For this review, take the finished solid that the model builds, in its own axes (mm). A direction names the side the tool comes from. Give positions to 0.01 mm unless a question says otherwise; leave off trailing zeros. Order: outer loops, then holes, each group sorted by start corner. A loop starts at its lowest first (then second) coordinate and runs counter-clockwise, first axis right, second up. Notation, with made-up numbers: M 63,-23 L 81,-23 A29 ccw 81,-3 Z; hole C 6.5,-8 d1. An arc over 180 degrees is marked long. Use CSV: the item, a comma, the result in double quotes. Start each with the question number.
(1) Wall thickness on L1, parallel to X at y = -6.4, z = 8; L2, parallel to X at y = 14.6, z = 88; L3, parallel to Z at x = -3.25, y = 1.5: over which ranges is each line inside the solid? List them lowest first. Write a range as from..to.
(2) Draft analysis for pull direction X (two halves, no side actions). For faces 6 (the face through (8.936, 12.535, 96.741)), 7 (the face through (-5.582, 11.521, 94.474)), 8 (the face through (-2, -7.5, 10)), state which applies: pulls with the +X half, pulls with the -X half, needs draft (parallel to the pull), parting line crosses it, or undercut.
(3) Tool access review of faces 1 (the face through (3, -2, 75.5)), 2 (the face through (0.1, 12, 85.5)), 3 (the face through (4.61, -5.34, 7.39)), 4 (the face through (1.5, 5, 81)), 5 (the face through (-0.2, 10.2, 70.5)): name each direction out of +Z, -Z, +X, -X, +Y, -Y from which nothing blocks a thin tool from reaching the whole face with its end or side.
(4) Clearance check with flat-ended pins moving along their axes: P1, Ø5, axis at y = 3.5, z = 13, coming from the +X side; P2, Ø1, axis at x = -9.5, z = 70.5, coming from the -Y side; P3, Ø1, axis at y = -6.5, z = 77, coming from the +X side; P4, Ø12.5, axis at x = -3.5, y = 7, coming from the -Z side. State where each tip first meets the part, or that it passes through.
(5) Consider section A-A (z = 8). Write out the cut boundary in (x, y).
(6) Consider section B-B (y = 0). Write out the cut boundary in (x, z).
```python
from build123d import *

# Parameters (mm, degrees)
SKETCH1_R                           = 5
BOSS_EXTRUDE1_DEPTH                 = 70.5
SKETCH3_W                           = 25
SKETCH3_H                           = 30
BOSS_EXTRUDE3_DEPTH                 = 5
SKETCH4_W                           = 25
SKETCH4_H                           = 5
BOSS_EXTRUDE4_DEPTH                 = 25
FILLET3_R                           = 12.5
CUT_EXTRUDE1_REACH                  = 107.624
SKETCH6_R                           = 1.65
SKETCH6_3_R                         = 10
SKETCH6_3_R_2                       = 1.65
SKETCH6_3_R_3                       = 2.5
CUT_EXTRUDE2_DEPTH                  = 2
SKETCH6_4_R                         = 2.5
CUT_EXTRUDE3_DEPTH                  = 4
FILLET4_R                           = 5
CUT_EXTRUDE4_REACH                  = 104.379
CUT_EXTRUDE4_END_RADIUS             = 5
SKETCH7_R                           = 2.65
CUT_EXTRUDE4_DIRECTION_2_REACH      = 104.379
CUT_EXTRUDE4_DIRECTION_2_END_RADIUS = 5
BOSS_EXTRUDE6_DEPTH                 = 7.5
BOSS_EXTRUDE6_DEPTH_BACK            = 7.5
SKETCH7_3_R                         = 4.65
SKETCH7_3_R_2                       = 2.65
BOSS_EXTRUDE7_DEPTH                 = 1.5
BOSS_EXTRUDE7_DEPTH_BACK            = 1.5


with BuildPart() as part:
    # Sketch1 → Boss-Extrude1 (new body)
    with BuildSketch(Plane(origin=(0, 0, 0), x_dir=(0, 1, 0), z_dir=(0, 0, 1))):
        with Locations(Location((0, 0, 0), (0, 0, 270))):
            Circle(SKETCH1_R)
    extrude(amount=BOSS_EXTRUDE1_DEPTH)

    # Sketch3 → Boss-Extrude3 (add)
    with BuildSketch(Plane.XY.offset(70.5)):
        Rectangle(SKETCH3_W, SKETCH3_H)
    extrude(amount=BOSS_EXTRUDE3_DEPTH)

    # Sketch4 → Boss-Extrude4 (add)
    with BuildSketch(Plane.XY.offset(75.5)):
        with Locations((0, 12.5)):
            Rectangle(SKETCH4_W, SKETCH4_H)
    extrude(amount=BOSS_EXTRUDE4_DEPTH)

    # Fillet3
    fillet3_edges = [part.edges().sort_by_distance(p)[0] for p in [
        (12.5, 12.5, 100.5),
        (-12.5, 12.5, 100.5),
        (-12.5, -15, 73),
        (12.5, -15, 73),
    ]]
    fillet(fillet3_edges, radius=FILLET3_R - 0.0001)  # a hair under: the kernel refuses the full size

    # Sketch6 → Cut-Extrude1 (cut, up to next)
    with BuildSketch(Plane(origin=(0, 15, 0), x_dir=(-1, 0, 0), z_dir=(0, 1, 0)), mode=Mode.PRIVATE) as cut_extrude1_sk1:
        with Locations(Location((-4.949747468, 92.949747468, 0), (0, 0, 90))):
            Circle(SKETCH6_R)
    cut_extrude1_tool1 = extrude(cut_extrude1_sk1.sketch, amount=-CUT_EXTRUDE1_REACH, mode=Mode.PRIVATE) & part.part
    # Sketch6 → Cut-Extrude1 (cut, up to next)
    with BuildSketch(Plane(origin=(0, 15, 0), x_dir=(-1, 0, 0), z_dir=(0, 1, 0)), mode=Mode.PRIVATE) as cut_extrude1_sk2:
        with Locations(Location((4.949747468, 92.949747468, 0), (0, 0, 90))):
            Circle(SKETCH6_R)
    cut_extrude1_tool2 = extrude(cut_extrude1_sk2.sketch, amount=-CUT_EXTRUDE1_REACH, mode=Mode.PRIVATE) & part.part
    # Sketch6 → Cut-Extrude1 (cut, up to next)
    with BuildSketch(Plane(origin=(0, 15, 0), x_dir=(-1, 0, 0), z_dir=(0, 1, 0)), mode=Mode.PRIVATE) as cut_extrude1_sk3:
        with Locations(Location((-4.949747468, 83.050252532, 0), (0, 0, 90))):
            Circle(SKETCH6_R)
    cut_extrude1_tool3 = extrude(cut_extrude1_sk3.sketch, amount=-CUT_EXTRUDE1_REACH, mode=Mode.PRIVATE) & part.part
    # Sketch6 → Cut-Extrude1 (cut, up to next)
    with BuildSketch(Plane(origin=(0, 15, 0), x_dir=(-1, 0, 0), z_dir=(0, 1, 0)), mode=Mode.PRIVATE) as cut_extrude1_sk4:
        with Locations(Location((4.949747468, 83.050252532, 0), (0, 0, 90))):
            Circle(SKETCH6_R)
    cut_extrude1_tool4 = extrude(cut_extrude1_sk4.sketch, amount=-CUT_EXTRUDE1_REACH, mode=Mode.PRIVATE) & part.part
    add(cut_extrude1_tool1.solids().sort_by_distance((4.949747, 15, 92.949747))[0], mode=Mode.SUBTRACT)
    add(cut_extrude1_tool2.solids().sort_by_distance((-4.949747, 15, 92.949747))[0], mode=Mode.SUBTRACT)
    add(cut_extrude1_tool3.solids().sort_by_distance((4.949747, 15, 83.050253))[0], mode=Mode.SUBTRACT)
    add(cut_extrude1_tool4.solids().sort_by_distance((-4.949747, 15, 83.050253))[0], mode=Mode.SUBTRACT)

    # Sketch6<3> → Cut-Extrude2 (cut)
    # profile 1 of 6: a face of its own
    with BuildSketch(Plane(origin=(0, 15, 0), x_dir=(-1, 0, 0), z_dir=(0, 1, 0))):
        with Locations(Location((0, 88, 0), (0, 0, 90))):
            Circle(SKETCH6_3_R)
        with Locations(Location((4.949747468, 83.050252532, 0), (0, 0, 90))):
            Circle(SKETCH6_3_R_2, mode=Mode.SUBTRACT)
        with Locations(Location((-4.949747468, 83.050252532, 0), (0, 0, 90))):
            Circle(SKETCH6_3_R_2, mode=Mode.SUBTRACT)
        with Locations(Location((4.949747468, 92.949747468, 0), (0, 0, 90))):
            Circle(SKETCH6_3_R_2, mode=Mode.SUBTRACT)
        with Locations(Location((-4.949747468, 92.949747468, 0), (0, 0, 90))):
            Circle(SKETCH6_3_R_2, mode=Mode.SUBTRACT)
        with Locations((0, 88)):
            Circle(SKETCH6_3_R_3, mode=Mode.SUBTRACT)
    # profile 2 of 6: a face of its own
    with BuildSketch(Plane(origin=(0, 15, 0), x_dir=(-1, 0, 0), z_dir=(0, 1, 0))):
        with Locations(Location((4.949747468, 92.949747468, 0), (0, 0, 90))):
            Circle(SKETCH6_3_R_2)
    # profile 3 of 6: a face of its own
    with BuildSketch(Plane(origin=(0, 15, 0), x_dir=(-1, 0, 0), z_dir=(0, 1, 0))):
        with Locations(Location((-4.949747468, 92.949747468, 0), (0, 0, 90))):
            Circle(SKETCH6_3_R_2)
    # profile 4 of 6: a face of its own
    with BuildSketch(Plane(origin=(0, 15, 0), x_dir=(-1, 0, 0), z_dir=(0, 1, 0))):
        with Locations(Location((-4.949747468, 83.050252532, 0), (0, 0, 90))):
            Circle(SKETCH6_3_R_2)
    # profile 5 of 6: a face of its own
    with BuildSketch(Plane(origin=(0, 15, 0), x_dir=(-1, 0, 0), z_dir=(0, 1, 0))):
        with Locations(Location((4.949747468, 83.050252532, 0), (0, 0, 90))):
            Circle(SKETCH6_3_R_2)
    # profile 6 of 6: a face of its own
    with BuildSketch(Plane(origin=(0, 15, 0), x_dir=(-1, 0, 0), z_dir=(0, 1, 0))):
        with Locations((0, 88)):
            Circle(SKETCH6_3_R_3)
    extrude(amount=-CUT_EXTRUDE2_DEPTH, mode=Mode.SUBTRACT)

    # Sketch6<4> → Cut-Extrude3 (cut)
    with BuildSketch(Plane(origin=(0, 15, 0), x_dir=(-1, 0, 0), z_dir=(0, 1, 0))):
        with Locations(Location((0, 88, 0), (0, 0, 90))):
            Circle(SKETCH6_4_R)
    extrude(amount=-CUT_EXTRUDE3_DEPTH, mode=Mode.SUBTRACT)

    # Fillet4
    fillet4_edges = [part.edges().sort_by_distance(p)[0] for p in [
        (-5, 0, 70.5),
    ]]
    fillet(fillet4_edges, radius=FILLET4_R)

    # Cut-Extrude4: up to this cylinder (the profile starts inside it)
    cut_extrude4_end = Plane(origin=(0, 0, 8), z_dir=(0, 0, -1)) * Cylinder(CUT_EXTRUDE4_END_RADIUS, 219.758, mode=Mode.PRIVATE)
    # Sketch7 → Cut-Extrude4 (cut, up to the surface)
    with BuildSketch(Plane(origin=(0, 0, 0), x_dir=(-1, 0, 0), z_dir=(0, 1, 0)), mode=Mode.PRIVATE) as cut_extrude4_sk1:
        with Locations(Location((0, 8, 0), (0, 0, 270))):
            Circle(SKETCH7_R)
    cut_extrude4_tool1 = extrude(cut_extrude4_sk1.sketch, amount=-CUT_EXTRUDE4_REACH, mode=Mode.PRIVATE) & cut_extrude4_end
    add(cut_extrude4_tool1.solids().sort_by_distance((0, 0, 8))[0], mode=Mode.SUBTRACT)

    # Cut-Extrude4 direction 2: up to this cylinder (the profile starts inside it)
    cut_extrude4_direction_2_end = Plane(origin=(0, 0, 8), z_dir=(0, 0, -1)) * Cylinder(CUT_EXTRUDE4_DIRECTION_2_END_RADIUS, 219.758, mode=Mode.PRIVATE)
    # Sketch7 → Cut-Extrude4 direction 2 (cut, up to the surface)
    with BuildSketch(Plane(origin=(0, 0, 0), x_dir=(-1, 0, 0), z_dir=(0, 1, 0)), mode=Mode.PRIVATE) as cut_extrude4_direction_2_sk1:
        with Locations(Location((0, 8, 0), (0, 0, 270))):
            Circle(SKETCH7_R)
    cut_extrude4_direction_2_tool1 = extrude(cut_extrude4_direction_2_sk1.sketch, amount=CUT_EXTRUDE4_DIRECTION_2_REACH, mode=Mode.PRIVATE) & cut_extrude4_direction_2_end
    add(cut_extrude4_direction_2_tool1.solids().sort_by_distance((0, 0, 8))[0], mode=Mode.SUBTRACT)

    # Sketch7<3> → Boss-Extrude6 (add, two sides: drawn at the far end of the back side and taken through both)
    with BuildSketch(Plane(origin=(0, 0, 0), x_dir=(-1, 0, 0), z_dir=(0, 1, 0)).offset(-BOSS_EXTRUDE6_DEPTH_BACK)):
        with Locations(Location((0, 8, 0), (0, 0, 90))):
            Circle(SKETCH7_3_R)
        with Locations(Location((0, 8, 0), (0, 0, 270))):
            Circle(SKETCH7_3_R_2, mode=Mode.SUBTRACT)
    extrude(amount=BOSS_EXTRUDE6_DEPTH + BOSS_EXTRUDE6_DEPTH_BACK)

    # Sketch9 → Boss-Extrude7 (add, two sides: drawn at the far end of the back side and taken through both)
    with BuildSketch(Plane(origin=(0, 0, 0), x_dir=(0, -1, 0), z_dir=(-1, 0, 0)).offset(-BOSS_EXTRUDE7_DEPTH_BACK)):
        Polygon((-10, 94.25), (8.75, 75.5), (-10, 75.5), align=None)
    extrude(amount=BOSS_EXTRUDE7_DEPTH + BOSS_EXTRUDE7_DEPTH_BACK)


solid = part.part
```
Check result:
1,L1,"x = -4.65..-2.65, 2.65..4.65"
1,L2,"x = -12.5..-10, 10..12.5"
1,L3,"z = 0..75.5"
2,face 6,"pulls with the +X half"
2,face 7,"undercut"
2,face 8,"needs draft"
3,face 1,"+Z, -Y"
3,face 2,"+Y"
3,face 3,"-Y"
3,face 4,"+Z, +X, -Y"
3,face 5,"-Z"
4,P1,"stops at x = 4.9"
4,P2,"stops at y = -11.17"
4,P3,"stops at x = 1.5"
4,P4,"stops at z = 0"
5,outline,"M -4.65,-7.5 L -2.65,-7.5 L -2.65,7.5 L -4.65,7.5 L -4.65,1.84 A5 ccw -4.65,-1.84 Z; M 2.65,-7.5 L 4.65,-7.5 L 4.65,-1.84 A5 ccw 4.65,1.84 L 4.65,7.5 L 2.65,7.5 Z"
6,outline,"M -12.5,70.5 L -10,70.5 A5 cw -5,65.5 L -5,0 L 5,0 L 5,65.5 A5 cw 10,70.5 L 12.5,70.5 L 12.5,75.5 L 1.5,75.5 L 1.5,84.25 L -1.5,84.25 L -1.5,75.5 L -12.5,75.5 Z; hole C 0,8 d5.3"
